Work out the finished part from the listing and answer in its coordinate system (mm). Face numbers are marked on the shaded views. A direction names the side the tool comes from. Coordinates: 2 decimals unless noted, no trailing zeros. Loops run counter-clockwise (first coordinate to the right, second up) from the corner with the lowest first, then second, coordinate; pieces in that order, holes last. Notation, with made-up numbers: (40.25, 20) - (75.25, 20) arc R10 cw to (75.25, 27) - close; hole circle Ø6 at (73, 7.25). An arc over 180 degrees is marked (long way). Write each question's results on one line, items separated by ' | '. Start each with the question number.
Item 1: Section B-B, the plane y = 0 is taken. Write down the section's boundary in (x, z), plus the area to 3 significant figures.
Item 2: Each of these flat-tipped pins is pushed along its axis until it touches: pin 1 Ø17 at (x, y) = (-9, 11.5) entering from -Z; pin 2 Ø20 at (x, y) = (21.659, 0) entering from +Z. Where does it stop, or does it pass through?
Item 3: A tool of negligible diameter and unlimited length cuts with its end or side. For the marked faces 5 and 6, from which of +Z, -Z, +X, -X, +Y, -Y can it reach the whole face along a straight path? Write none if from no direction.
Item 4: Section C-C, the plane z = 9.25 is taken. Write down the section's boundary in (x, y).
Item 5: For a pull along Y with two mould halves and no side action, classify the marked faces 1, 2, 3 and 4 as +Y half, -Y half, draft (parallel to the pull), parting line (faces both ways), or undercut.
Item 6: Section A-A, the plane x = -21.66 is taken. Write down the section's boundary in (y, z).
Item 7: Section D-D, the plane y = -20 is taken. Write down the section's boundary in (x, z), plus the area to 3 significant figures.
Item 8: Consider probe 1 along X at (y, z) = (0, 17.6); probe 2 along Y at (x, z) = (-21.66, 17.95); probe 3 along Y at (x, z) = (0, 12.75). Determine where each line is inside the solid, lowest interval first. Write a range as [from, to].
from build123d import *

# Parameters (mm, degrees)
SKETCH_W        = 100
SKETCH_H        = 60
PAD_DEPTH       = 19
SKETCH001_W     = 96
SKETCH001_H     = 56
POCKET_DEPTH    = 17
SKETCH002_R     = 11.1
POCKET001_DEPTH = 20
SKETCH003_R     = 11.1
POCKET002_DEPTH = 20


with BuildPart() as part:
    # Sketch → Pad (new body)
    with BuildSketch(Plane.XY):
        Rectangle(SKETCH_W, SKETCH_H)
    extrude(amount=PAD_DEPTH)

    # Sketch001 → Pocket (cut)
    with BuildSketch(Plane.XY):
        Rectangle(SKETCH001_W, SKETCH001_H)
    extrude(amount=POCKET_DEPTH, mode=Mode.SUBTRACT)

    # Sketch002 → Pocket001 (cut)
    with BuildSketch(Plane.XY):
        with Locations((-21.66, 0)):
            Circle(SKETCH002_R)
    extrude(amount=POCKET001_DEPTH, mode=Mode.SUBTRACT)

    # Sketch003 → Pocket002 (cut)
    with BuildSketch(Plane.XY):
        with Locations((21.659, 0)):
            Circle(SKETCH003_R)
    extrude(amount=POCKET002_DEPTH, mode=Mode.SUBTRACT)


solid = part.part
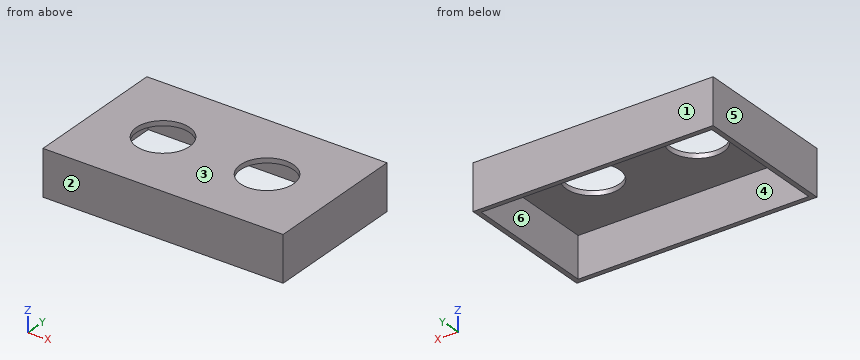
Answer key:
1) outline: (-50, 0) - (-48, 0) - (-48, 17) - (-32.76, 17) - (-32.76, 19) - (-50, 19) - close; (-10.56, 17) - (10.56, 17) - (10.56, 19) - (-10.56, 19) - close; (32.76, 17) - (48, 17) - (48, 0) - (50, 0) - (50, 19) - (32.76, 19) - close | area: 179 mm^2
2) pin 1: stops at z = 17 | pin 2: passes through
3) face 5: +Z, -Z, -X, +Y, -Y | face 6: -Z
4) outline: (-50, -30) - (50, -30) - (50, 30) - (-50, 30) - close; hole (-48, -28) - (48, -28) - (48, 28) - (-48, 28) - close
5) face 1: +Y half | face 2: -Y half | face 3: draft | face 4: undercut
6) outline: (-30, 0) - (-28, 0) - (-28, 17) - (-11.1, 17) - (-11.1, 19) - (-30, 19) - close; (11.1, 17) - (28, 17) - (28, 0) - (30, 0) - (30, 19) - (11.1, 19) - close
7) outline: (-50, 0) - (-48, 0) - (-48, 17) - (48, 17) - (48, 0) - (50, 0) - (50, 19) - (-50, 19) - close | area: 268 mm^2
8) probe 1: x = [-50, -32.76], [-10.56, 10.56], [32.76, 50] | probe 2: y = [-30, -11.1], [11.1, 30] | probe 3: y = [-30, -28], [28, 30]
